Build history of the part. All positions in model axes, mm. Round coordinates to 2 decimals unless told otherwise and drop trailing zeros. Loops run counter-clockwise (first coordinate to the right, second up) from the corner with the lowest first, then second, coordinate; pieces in that order, holes last. Notation, with made-up numbers: (50, 22.25) - (86, 22.25) arc R8 cw to (86, 37.25) - close; hole circle Ø6 at (-27.75, -36). An arc over 180 degrees is marked (long way). Use one line per item in the form item = value. Start each with the question number.
Q1. Saw through at A-A (y = 25). Give the cut face in (x, z), then the cut area to 3 significant figures.
Q2. Pin check, flat tips, straight feed: pin 1 (1.5 mm diameter, centred on y = -69.5, z = 2, fed in from -X); pin 2 (2.5 mm diameter, centred on y = -72, z = 2.5, fed in from +X); pin 3 (2.5 mm diameter, centred on x = 41, z = 2.5, fed in from -Y). Stop position of each tip, or through.
Q3. Saw through at B-B (x = -56). Give the cut face in (y, z).
Q4. Drill centre lines: line 1 (X direction, y = 36, z = 4.3); line 2 (Y direction, x = 58, z = 2.45); line 3 (X direction, y = -66.5, z = 4.35). Where is each one in solid material? Low to high.
Q5. Saw through at C-C (z = 2.55). Give the cut face in (x, y), then the cut area to 3 significant figures.
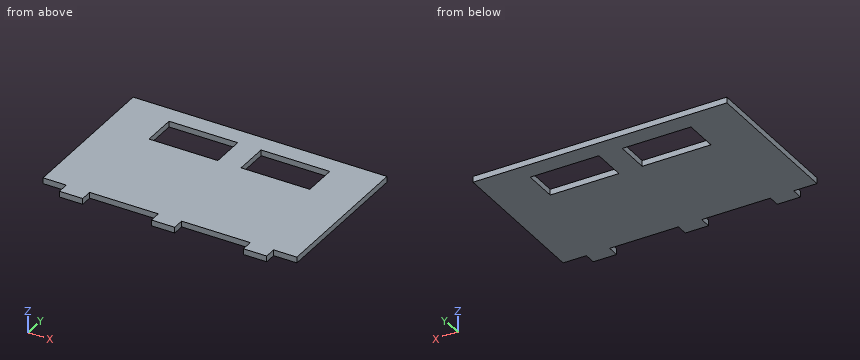
```python
from build123d import *

# Parameters (mm, degrees)
SKETCH1_W           = 218
SKETCH1_H           = 131
SKETCH1_W_2         = 59
SKETCH1_H_2         = 29
SKETCH1_W_3         = 20
SKETCH1_H_3         = 10
BOSS_EXTRUDE1_DEPTH = 5


with BuildPart() as part:
    # Sketch1 → Boss-Extrude1 (new body)
    with BuildSketch(Plane.XY):
        Rectangle(SKETCH1_W, SKETCH1_H)
        with Locations((39.5, 35.5)):
            Rectangle(SKETCH1_W_2, SKETCH1_H_2, mode=Mode.SUBTRACT)
        with Locations((-39.5, 35.5)):
            Rectangle(SKETCH1_W_2, SKETCH1_H_2, mode=Mode.SUBTRACT)
        with Locations((-79, -70.5)):
            Rectangle(SKETCH1_W_3, SKETCH1_H_3)
        with Locations((0, -70.5)):
            Rectangle(SKETCH1_W_3, SKETCH1_H_3)
        with Locations((79, -70.5)):
            Rectangle(SKETCH1_W_3, SKETCH1_H_3)
    extrude(amount=BOSS_EXTRUDE1_DEPTH)


solid = part.part
```
Report:
q1.outline = (-109, 0) - (-69, 0) - (-69, 5) - (-109, 5) - close; (-10, 0) - (10, 0) - (10, 5) - (-10, 5) - close; (69, 0) - (109, 0) - (109, 5) - (69, 5) - close
q1.area = 500 mm²
q2.pin_1 = -89
q2.pin_2 = 89
q2.pin_3 = -65.5
q3.outline = (-65.5, 0) - (21, 0) - (21, 5) - (-65.5, 5) - close; (50, 0) - (65.5, 0) - (65.5, 5) - (50, 5) - close
q4.line_1 = -109 to -69, -10 to 10, 69 to 109
q4.line_2 = -65.5 to 21, 50 to 65.5
q4.line_3 = -89 to -69, -10 to 10, 69 to 89
q5.outline = (-109, -65.5) - (-89, -65.5) - (-89, -75.5) - (-69, -75.5) - (-69, -65.5) - (-10, -65.5) - (-10, -75.5) - (10, -75.5) - (10, -65.5) - (69, -65.5) - (69, -75.5) - (89, -75.5) - (89, -65.5) - (109, -65.5) - (109, 65.5) - (-109, 65.5) - close; hole (-69, 21) - (-10, 21) - (-10, 50) - (-69, 50) - close; hole (10, 21) - (69, 21) - (69, 50) - (10, 50) - close
q5.area = 25,700 mm²
